Can you work these out from the model? Positions are in its coordinate system, mm. Face numbers are marked on the shaded views. Give positions to 0.01 mm unless a question says otherwise; leave off trailing zeros. Loops run counter-clockwise (first coordinate to the right, second up) from the corner with the lowest first, then second, coordinate; pieces in that order, holes last.
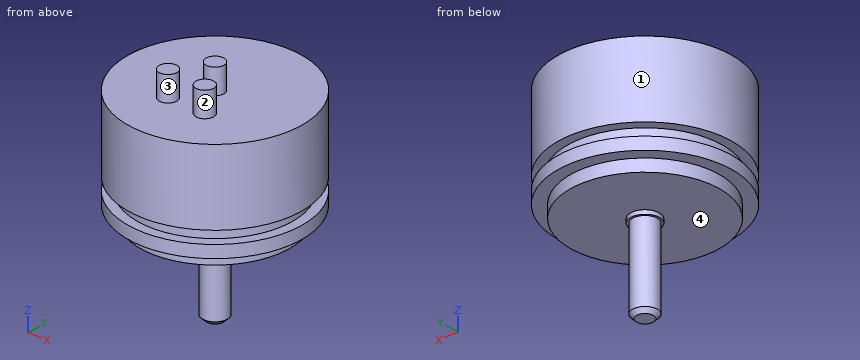
from build123d import *

# Parameters (mm, degrees)
SKETCH3_R           = 1.143
BOSS_EXTRUDE1_DEPTH = 3.175


with BuildPart() as part:
    # Sketch2 → Revolve2 (revolve)
    with BuildSketch(Plane(origin=(0, 0, 0), x_dir=(0, 0, -1), z_dir=(1, 0, 0)), mode=Mode.PRIVATE) as revolve2_sk:
        Polygon((-9.5504, 11.1125), (-9.5504, 0), (4.7244, 0), (4.7244, 1.83896), (4.7244, 9.525), (3.1496, 9.525), (3.1496, 11.1125), (1.5748, 11.1125), (1.5748, 9.906), (0, 9.906), (0, 11.1125), align=None)
        Polygon((4.7244, 1.83896), (4.7244, 0), (15.8496, 0), (15.8496, 1.07696), (15.3416, 1.58496), (5.2324, 1.58496), (5.2324, 1.83896), align=None)
    revolve(revolve2_sk.sketch.rotate(Axis((0, 0, 28.040799935), (0, 0, -1)), 90), axis=Axis((0, 0, 28.040799935), (0, 0, -1)))

    # Sketch3 → Boss-Extrude1 (add)
    with BuildSketch(Plane.XY.offset(9.5504)):
        Circle(SKETCH3_R)
        with Locations((-2.413, -4.179438599)):
            Circle(SKETCH3_R)
        with Locations((2.413, -4.179438599)):
            Circle(SKETCH3_R)
    extrude(amount=BOSS_EXTRUDE1_DEPTH)


solid = part.part
(1) Suppose I cut it at C-C on z = 3.25. List the corners of the cut face in (x, y) for me (1 decimal), plus the area to 3 significant figures.
Returned:
outline: circle Ø22.2 at (0, 0)
area: 388 mm2
(2) Thinking about a two-plate mould opening in X: for the marked faces 1, 2, 3 and 4, which applies, pulls with the +X half, pulls with the -X half, needs draft (parallel to the pull), parting line crosses it, or undercut?
Returned:
face 1: parting line crosses it
face 2: undercut
face 3: undercut
face 4: needs draft
(3) Will these pins go through, and if not, where does the flat tip stop? P1, Ø4, axis at x = -8, y = 5, coming from the -Z side; P2, Ø5, axis at x = 8, z = -6, coming from the +Y side; P3, Ø2, axis at x = 4.5, z = -5, coming from the -Y side.
Returned:
P1: stops at z = -4.72
P2: stops at y = 7.52
P3: stops at y = -8.84
(4) Suppose I cut it at D-D on y = 3.75. List the corners of the cut face in (x, z) for me.
Returned:
outline: (-10.46, -3.15) - (-8.76, -3.15) - (-8.76, -4.72) - (8.76, -4.72) - (8.76, -3.15) - (10.46, -3.15) - (10.46, -1.57) - (9.17, -1.57) - (9.17, 0) - (10.46, 0) - (10.46, 9.55) - (-10.46, 9.55) - (-10.46, 0) - (-9.17, 0) - (-9.17, -1.57) - (-10.46, -1.57) - close
(5) Please list where these lines run through material, in increasing order: probe 1 along Z at (x, y) = (7, -7.5); probe 2 along Z at (x, y) = (-6, 1.5); probe 3 along Z at (x, y) = (-8.25, -5).
Returned:
probe 1: z = -3.15 to -1.57, 0 to 9.55
probe 2: z = -4.72 to 9.55
probe 3: z = -3.15 to 9.55
